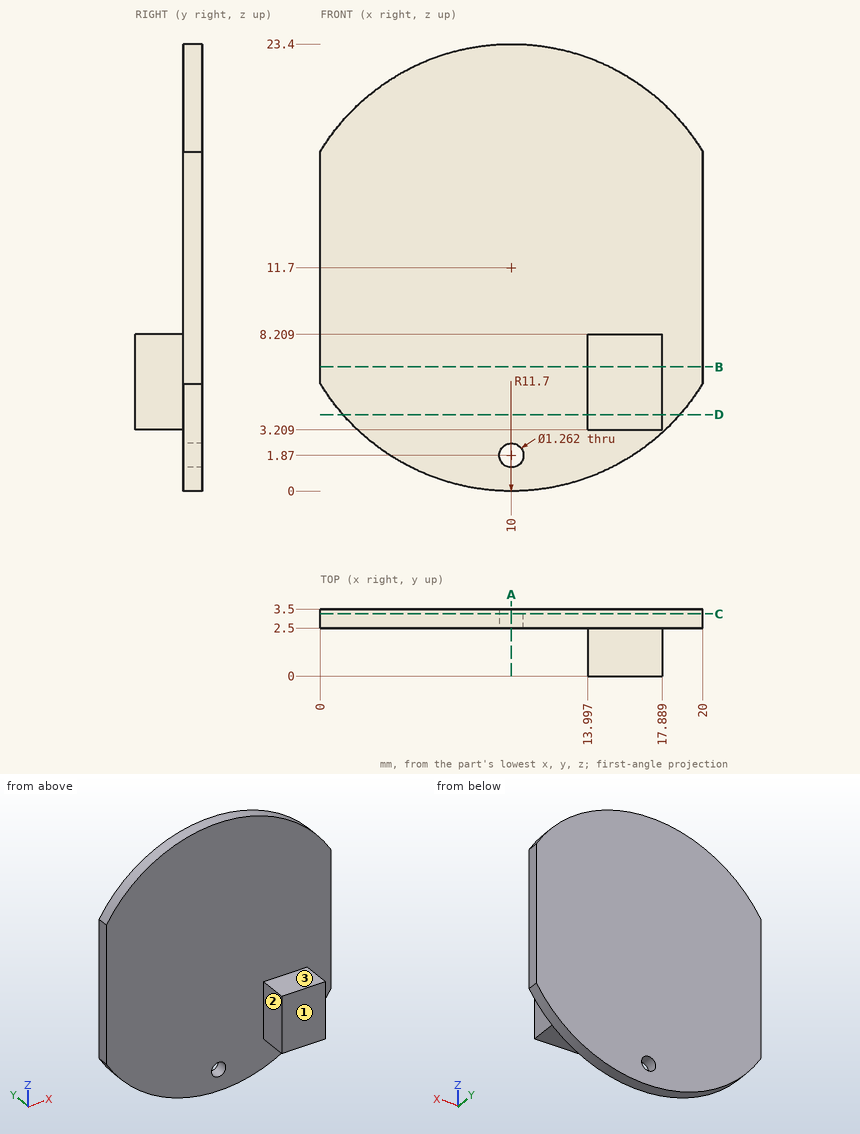
For this review, use the dimensioned drawing (mm, ordinates from the lowest corner) and the shaded views. A direction names the side the tool comes from. Coordinates: 2 decimals unless noted, no trailing zeros. Loops run counter-clockwise (first coordinate to the right, second up) from the corner with the lowest first, then second, coordinate; pieces in that order, holes last. Notation, with made-up numbers: (27.5, 2) -> (57.5, 2) arc R17 ccw to (57.5, 8) -> close; hole circle Ø2 at (-8.5, 52.25). An arc over 180 degrees is marked (long way). Use a Markdown table: item, result. Add a question column.
Item 1: We need section A-A, the plane x = 10. Write out the cut boundary in (y, z).
Item 2: We need section D-D, the plane z = 4. Write out the cut boundary in (x, y).
Item 3: Clearance check with flat-ended pins moving along their axes: P1, Ø0.8, axis at y = 1.5, z = 7, coming from the -X side; P2, Ø0.8, axis at x = 16.5, y = 1.5, coming from the -Z side; P3, Ø6, axis at x = 14.5, z = 13.5, coming from the -Y side. State where each tip first meets the part, or that it passes through.
Item 4: We need section C-C, the plane y = 3.25. Write out the cut boundary in (x, z).
Item 5: We need section B-B, the plane z = 6.5. Write out the cut boundary in (x, y).
Item 6: Wall thickness on L1, parallel to Z at x = 10, y = 2.9; L2, parallel to Z at x = 17, y = 1.45; L3, parallel to Y at x = 3.5, z = 3: over which ranges is each line inside the solid? List them lowest first. Write a range as from..to.
Item 7: Machinability: for the marked faces 1, 2 and 3, which of the approach directions +Z, -Z, +X, -X, +Y, -Y give a long, thin tool a straight path to every point of the face, cutting with its end or side? Answer none if there is none.
Numbers:
| question | item | result |
|---|---|---|
| 1 | outline | (2.5, 0) -> (3.5, 0) -> (3.5, 1.24) -> (2.5, 1.24) -> close; (2.5, 2.5) -> (3.5, 2.5) -> (3.5, 23.4) -> (2.5, 23.4) -> close |
| 2 | outline | (1.19, 2.5) -> (14, 2.5) -> (14, 0) -> (17.89, 0) -> (17.89, 2.5) -> (18.81, 2.5) -> (18.81, 3.5) -> (1.19, 3.5) -> close |
| 3 | P1 | stops at x = 14 |
| 3 | P2 | stops at z = 3.21 |
| 3 | P3 | stops at y = 2.5 |
| 4 | outline | (0, 5.63) arc R11.7 ccw to (20, 5.63) -> (20, 17.77) arc R11.7 ccw to (0, 17.77) -> close; hole circle Ø1.26 at (10, 1.87) |
| 5 | outline | (0, 2.5) -> (14, 2.5) -> (14, 0) -> (17.89, 0) -> (17.89, 2.5) -> (20, 2.5) -> (20, 3.5) -> (0, 3.5) -> close |
| 6 | L1 | z = 0..1.24, 2.5..23.4 |
| 6 | L2 | z = 3.21..8.21 |
| 6 | L3 | y = 2.5..3.5 |
| 7 | face 1 | +Z, -Z, +X, -X, -Y |
| 7 | face 2 | +Z, -Z, -X, -Y |
| 7 | face 3 | +Z, +X, -X, -Y |
